Input: dimensioned drawing with shaded views. Units: mm. Origin: part minimum x, y, z. A direction names the side the tool comes from. Give positions to 0.01 mm unless a question says otherwise; leave off trailing zeros. Order: outer loops, then holes, each group sorted by start corner. A loop starts at its lowest first (then second) coordinate and runs counter-clockwise, first axis right, second up. Notation, with made-up numbers: (41.25, 19.25) -> (62.25, 19.25) arc R28 cw to (62.25, 56.25) -> close; hole circle Ø7 at (76.25, -6). An arc over 180 degrees is marked (long way). One line per question, with ' | ' between items. Start each with the question number.
(1) Mould query, pull axis X, two halves, no side actions, for the marked faces 3, 4 and 5. Classes: +X half, -X half, draft (parallel to the pull), parting line (faces both ways), or undercut.
(2) Set-up query: the marked faces 1 and 2. Return all of +Z, -Z, +X, -X, +Y, -Y with unobstructed straight access to the full face (end or side cutting, diameter ignored); none if empty.
(3) Section B-B (z = 23). Return loops of the section in (x, y), then the cut area to 3 significant figures.
(4) Section A-A (y = 28). State how many separate pieces and enclosed holes the cut face has, then the cut area to 3 significant figures.
(5) Section C-C (z = 13.5). Return loops of the section in (x, y).
(6) Ray query, L1, parallel to X at y = 28, z = 8.5; L2, parallel to Z at x = 79, y = 36; L3, parallel to Z at x = 30, y = 21 (1 decimal). Return the intervals inside material, ascending.
(7) Section D-D (x = 48). Return loops of the section in (y, z), then the cut area to 3 significant figures.
(8) First-contact query: pin 1 Ø6 at (x, y) = (89, 38) entering from -Z; pin 2 Ø6 at (x, z) = (14.5, 30.5) entering from -Y; pin 3 Ø10.5 at (x, y) = (89.5, 28.5) entering from +Z; pin 4 Ø6 at (y, z) = (31.5, 17) entering from -X. Flat tips, straight axial feed; report the tip coordinate or a pass-through.
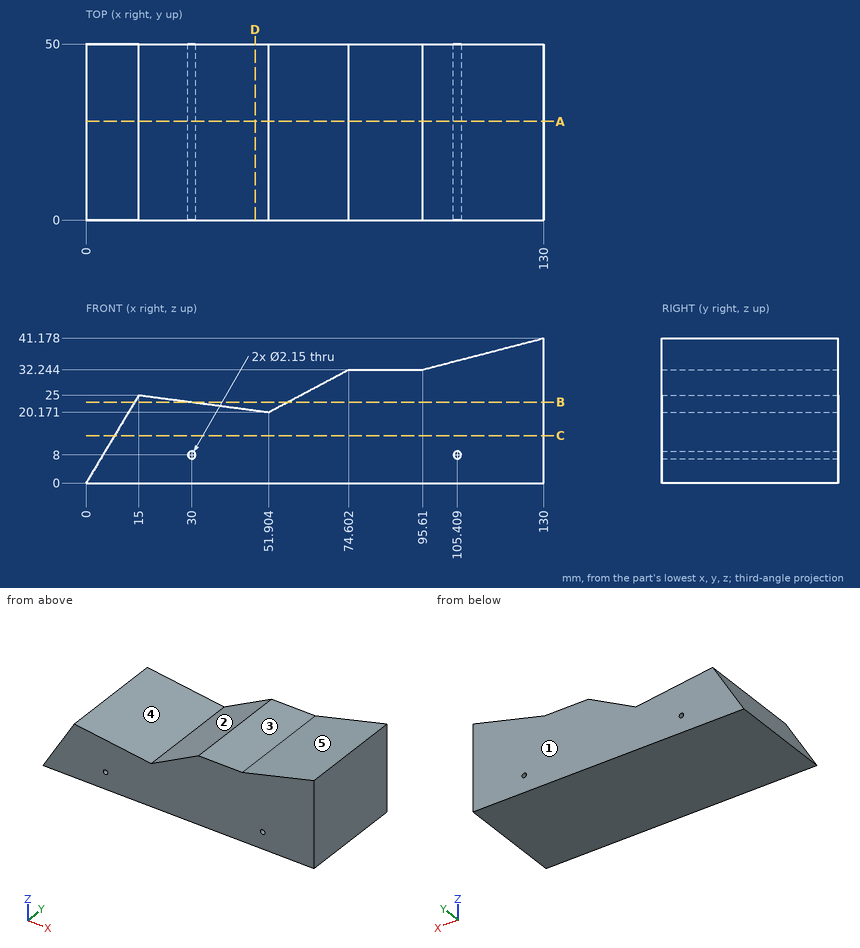
Response:
1) face 3: draft | face 4: undercut | face 5: -X half
2) face 1: +Z, -Z, +X, -X, +Y | face 2: +Z, +Y, -Y
3) outline: (13.8, 0) -> (30.28, 0) -> (30.28, 50) -> (13.8, 50) -> close; (57.22, 0) -> (130, 0) -> (130, 50) -> (57.22, 50) -> close | area: 4,460 mm^2
4) separate pieces: 1 | enclosed holes: 2 | area: 3,550 mm^2
5) outline: (8.1, 0) -> (130, 0) -> (130, 50) -> (8.1, 50) -> close
6) L1: x = 5.1 to 29.05, 30.95 to 104.46, 106.36 to 130 | L2: z = 0 to 32.24 | L3: z = 0 to 6.9, 9.1 to 23
7) outline: (0, 0) -> (50, 0) -> (50, 20.68) -> (0, 20.68) -> close | area: 1,030 mm^2
8) pin 1: stops at z = 0 | pin 2: passes through | pin 3: stops at z = 32.24 | pin 4: stops at x = 8.4
